from build123d import *

# Parameters (mm, degrees)
SKETCH1_R          = 11.8999
BODY_DEPTH         = 11.303
SKETCH2_R          = 4.7625
BUSHING_DEPTH      = 9.525
SKETCH3_W          = 1.5748
SKETCH3_H          = 4.1656
MOUNT_TAB_DEPTH    = 4.064
SKETCH4_R          = 3.175
CUT_EXTRUDE1_DEPTH = 9.525
SKETCH5_W          = 20.4216
SKETCH5_H          = 6.3754
BOARD_DEPTH        = 5.08


with BuildPart() as part:
    # Sketch1 → Body (new body)
    with BuildSketch(Plane.XY):
        Circle(SKETCH1_R)
    extrude(amount=-BODY_DEPTH)

    # Sketch2 → bushing (add)
    with BuildSketch(Plane.XY):
        Circle(SKETCH2_R)
    extrude(amount=BUSHING_DEPTH)

    # Sketch3 → mount tab (add)
    with BuildSketch(Plane.XY):
        with Locations((-11.2014, 0)):
            Rectangle(SKETCH3_W, SKETCH3_H)
        with Locations((11.2014, 0)):
            Rectangle(SKETCH3_W, SKETCH3_H)
    extrude(amount=MOUNT_TAB_DEPTH)

    # Sketch4 → Cut-Extrude1 (cut)
    with BuildSketch(Plane.XY.offset(9.525)):
        Circle(SKETCH4_R)
    extrude(amount=-CUT_EXTRUDE1_DEPTH, mode=Mode.SUBTRACT)

    # Sketch5 → board (add)
    with BuildSketch(Plane.XY):
        with Locations((0, -11.8999)):
            Rectangle(SKETCH5_W, SKETCH5_H)
    extrude(amount=-BOARD_DEPTH)


solid = part.part
The listing builds one solid part. Answer for the finished solid, in the listing's coordinates (mm). A direction names the side the tool comes from. Give positions to 0.01 mm unless a question says otherwise; leave off trailing zeros. Loops run counter-clockwise (first coordinate to the right, second up) from the corner with the lowest first, then second, coordinate; pieces in that order, holes last.
Item 1: A tool of negligible diameter and unlimited length cuts with its end or side. For faces 1 (the flat face through (-11, 0, 4.064)), 2 (the flat face through (10.414, 0, 2)), 3 (the flat face through (-11, 2.083, 2)), 4 (the flat face through (11, -2.083, 2)), 5 (the flat face through (-10.211, -12, -3)), from which of +Z, -Z, +X, -X, +Y, -Y can it reach the whole face along a straight path? Write none if from no direction.
Derived:
face 1: +Z, -X, +Y, -Y
face 2: +Z, +Y, -Y
face 3: +Z, -X, +Y
face 4: +Z, +X, -Y
face 5: +Z, -Z, -X, -Y
Item 2: A cutting plane is placed at A-A (x = 0). Give the vertices of the cut face in (y, z) (1 decimal).
Derived:
outline: (-15.1, -5.1) - (-11.9, -5.1) - (-11.9, -11.3) - (11.9, -11.3) - (11.9, 0) - (4.8, 0) - (4.8, 9.5) - (3.2, 9.5) - (3.2, 0) - (-3.2, 0) - (-3.2, 9.5) - (-4.8, 9.5) - (-4.8, 0) - (-15.1, 0) - close
Item 3: Determine the mould class of faces 6 (the flat face through (-10.414, 0, 2)), 7 (the flat face through (-11.989, 0, 2)), 8 (the cylindrical face through (-0.69, -3.1, 4.83)), 9 (the flat face through (-11, -2.083, 2)) for opening direction X: +X half, -X half, draft (parallel to the pull), parting line (faces both ways), or undercut.
Derived:
face 6: undercut
face 7: -X half
face 8: undercut
face 9: draft
Item 4: Each of these flat-tipped pins is pushed along its axis until it touches: pin 1 Ø1.5 at (y, z) = (-13, -2) entering from +X; pin 2 Ø0.8 at (x, z) = (-11, 2.5) entering from -Y; pin 3 Ø1.3 at (x, y) = (-11.5, 0) entering from +Z. Where does it stop, or does it pass through?
Derived:
pin 1: stops at x = 10.21
pin 2: stops at y = -2.08
pin 3: stops at z = 4.06
Item 5: A cutting plane is placed at B-B (y = -9.25). Give the vertices of the cut face in (x, z).
Derived:
outline: (-10.21, -5.08) - (-7.49, -5.08) - (-7.49, -11.3) - (7.49, -11.3) - (7.49, -5.08) - (10.21, -5.08) - (10.21, 0) - (-10.21, 0) - close
Item 6: A cutting plane is placed at C-C (z = -6.25). Give the vertices of the cut face in (x, y).
Derived:
outline: circle Ø23.8 at (0, 0)
Item 7: Find the intervals of material crossed by line 1 along Y through (x, z) = (0, 5.5) (1 decimal); line 2 along Z through (x, y) = (-2, 0); line 3 along Y through (x, z) = (2.75, 1.75), in increasing order.
Derived:
line 1: y = -4.8 to -3.2, 3.2 to 4.8
line 2: z = -11.3 to 0
line 3: y = -3.89 to -1.59, 1.59 to 3.89
